The listing builds one solid part. Answer for the finished solid, in the listing's coordinates (mm). A direction names the side the tool comes from. Give positions to 0.01 mm unless a question says otherwise; leave off trailing zeros. Order: outer loops, then holes, each group sorted by start corner. A loop starts at its lowest first (then second) coordinate and runs counter-clockwise, first axis right, second up.
```python
from build123d import *

# Parameters (mm, degrees)
SKETCH1_R           = 3
BOSS_EXTRUDE1_DEPTH = 25
SKETCH1_3_W         = 11
SKETCH1_3_H         = 10
SKETCH1_3_R         = 3
BOSS_EXTRUDE2_DEPTH = 8
FILLET1_R           = 0.6


with BuildPart() as part:
    # Sketch1 → Boss-Extrude1 (new body)
    with BuildSketch(Plane(origin=(0, 0, 0), x_dir=(1, 0, 0), z_dir=(0, 1, 0))):
        with Locations(Location((1.6, 0, 0), (0, 0, 270))):
            Circle(SKETCH1_R)
    extrude(amount=BOSS_EXTRUDE1_DEPTH)

    # Sketch1_3 → Boss-Extrude2 (add)
    with BuildSketch(Plane(origin=(0, 0, 0), x_dir=(1, 0, 0), z_dir=(0, 1, 0))):
        Rectangle(SKETCH1_3_W, SKETCH1_3_H)
        with Locations(Location((1.6, 0, 0), (0, 0, 90))):
            Circle(SKETCH1_3_R, mode=Mode.SUBTRACT)
    extrude(amount=BOSS_EXTRUDE2_DEPTH)

    # Fillet1
    fillet1_edges = [part.edges().sort_by_distance(p)[0] for p in [
        (1.6, 25, -3),
    ]]
    fillet(fillet1_edges, radius=FILLET1_R)


solid = part.part
```
1) A tool of negligible diameter and unlimited length cuts with its end or side. For faces 1 (the cylindrical face through (2.5, 16.09, 2.86)), 2 (the flat face through (-5.5, 4, 0)), from which of +Z, -Z, +X, -X, +Y, -Y can it reach the whole face along a straight path? Write none if from no direction.
Geometry says:
face 1: +Y
face 2: +Z, -Z, -X, +Y, -Y
2) Straight lines are drawn through the part: probe 1 along Y at (x, z) = (-4.25, 4.25); probe 2 along Z at (x, y) = (1.5, 12); probe 3 along X at (y, z) = (17.25, -1). For each, find the intervals that lie inside material, in ascending order.
Geometry says:
probe 1: y = 0 to 8
probe 2: z = -3 to 3
probe 3: x = -1.23 to 4.43
3) Find section C-C (y = 9.75). Write down the section's boundary in (x, z).
Geometry says:
outline: circle Ø6 at (1.6, 0)
4) Find section B-B (x = 1.6). Write down the section's boundary in (y, z).
Geometry says:
outline: (0, -5) - (8, -5) - (8, -3) - (24.4, -3) arc R0.6 ccw to (25, -2.4) - (25, 2.4) arc R0.6 ccw to (24.4, 3) - (8, 3) - (8, 5) - (0, 5) - close
5) Find section D-D (x = -3.5). Write down the section's boundary in (y, z).
Geometry says:
outline: (0, -5) - (8, -5) - (8, 5) - (0, 5) - close
6) Given P1, Ø6, axis at y = 20, z = 2.5, coming from the +X side, flat-ended and moving along its own axis, determine where the tip first touches the part or whether it passes through.
Geometry says:
P1: stops at x = 4.6
7) Find section A-A (z = 0). Write down the section's boundary in (x, y).
Geometry says:
outline: (-5.5, 0) - (5.5, 0) - (5.5, 8) - (4.6, 8) - (4.6, 24.4) arc R0.6 ccw to (4, 25) - (-0.8, 25) arc R0.6 ccw to (-1.4, 24.4) - (-1.4, 8) - (-5.5, 8) - close
